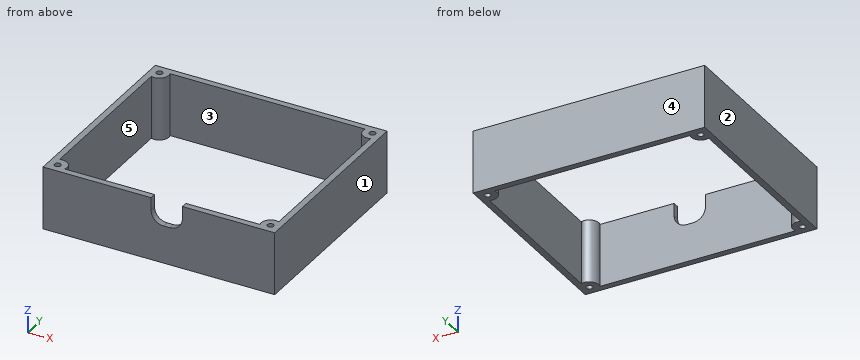
```python
from build123d import *

# Parameters (mm, degrees)
BOX010_W          = 10
BOX010_H          = 10
BOX010_DEPTH      = 10
FILLET001_R       = 4
BOX008_W          = 70
BOX008_H          = 60
BOX008_DEPTH      = 20
BOX007_W          = 74
BOX007_H          = 64
BOX007_DEPTH      = 20
CYLINDER007_R     = 1
CYLINDER007_DEPTH = 20
CYLINDER006_R     = 3
CYLINDER006_DEPTH = 20
ARRAY004_X_COUNT  = 2
ARRAY004_X_PITCH  = 68
ARRAY004_Y_COUNT  = 2
ARRAY004_Y_PITCH  = 58


with BuildPart() as fillet001:
    # Box010 → Box010 (new body)
    with BuildSketch(Plane(origin=(34.5, -4.5, 15), x_dir=(1, 0, 0), z_dir=(0, 0, 1))):
        with Locations((5, 5)):
            Rectangle(BOX010_W, BOX010_H)
    extrude(amount=BOX010_DEPTH)

    # Fillet001
    fillet001_edges = [fillet001.edges().sort_by_distance(p)[0] for p in [
        (34.5, 0.5, 15),
        (44.5, 0.5, 15),
    ]]
    fillet(fillet001_edges, radius=FILLET001_R)


with BuildPart() as wall_inner_extraction:
    # Box008 → Box008 (new body)
    with BuildSketch(Plane(origin=(2, 2, 0), x_dir=(1, 0, 0), z_dir=(0, 0, 1))):
        with Locations((35, 30)):
            Rectangle(BOX008_W, BOX008_H)
    extrude(amount=BOX008_DEPTH)


with BuildPart() as wall_box_cut:
    # Box007 → Box007 (new body)
    with BuildSketch(Plane.XY):
        with Locations((37, 32)):
            Rectangle(BOX007_W, BOX007_H)
    extrude(amount=BOX007_DEPTH)

    # Cut004: cut wall inner extraction
    add(wall_inner_extraction.part, mode=Mode.SUBTRACT)


with BuildPart() as wall_box_hole:
    # Cylinder007 → Cylinder007 (new body)
    with BuildSketch(Plane.XY):
        Circle(CYLINDER007_R)
    extrude(amount=CYLINDER007_DEPTH)


with BuildPart() as wall_fusion_cut:
    # Cylinder006 → Cylinder006 (new body)
    with BuildSketch(Plane.XY):
        Circle(CYLINDER006_R)
    extrude(amount=CYLINDER006_DEPTH)

    # Cut005: cut wall box hole
    add(wall_box_hole.part, mode=Mode.SUBTRACT)


with BuildPart() as wall_fusion_cut_1:
    # Cut005 placement: moved
    add(wall_fusion_cut.part.moved(Location((3, 3, 0))))

    # Array004 X: wall fusion cut ×2


with BuildPart() as wall_fusion_cut_2:
    add(wall_fusion_cut_1.part)
    with Locations(*[(i * ARRAY004_X_PITCH, 0, 0) for i in range(1, ARRAY004_X_COUNT)]):
        add(wall_fusion_cut_1.part)

    # Array004 Y: wall fusion cut ×2


with BuildPart() as wall_fusion_cut_3:
    add(wall_fusion_cut_2.part)
    with Locations(*[(0, i * ARRAY004_Y_PITCH, 0) for i in range(1, ARRAY004_Y_COUNT)]):
        add(wall_fusion_cut_2.part)

    # Fusion003: union wall box cut
    add(wall_box_cut.part)


with BuildPart() as wall_fusion_cut_4:
    # Fusion003 placement: moved
    add(wall_fusion_cut_3.part.moved(Location((0, 0, 3))))

    # Cut007: cut Fillet001
    add(fillet001.part, mode=Mode.SUBTRACT)


solid = wall_fusion_cut_4.part
```
Source: CAD feature listing. Evaluate the final solid. Frame: model axes, mm. Face numbers are marked on the shaded views. A direction names the side the tool comes from. Give positions to 0.01 mm unless a question says otherwise; leave off trailing zeros. Write each loop counter-clockwise with the first axis right and the second up, starting at its lowest first coordinate (ties: lowest second). Pieces come first, ordered by that corner, then holes.
1. Section query A-A (x = 16). Return the cut outline in (y, z).
2. Material intervals for line 1 along Y through (x, z) = (71, 13); line 2 along X through (y, z) = (3, 12.75); line 3 along Y through (x, z) = (22.5, 20.5), sorted ascending.
3. Section query B-B (y = 61). Return the cut outline in (x, z).
4. Access query for the marked faces 4 and 5. Directions: +Z, -Z, +X, -X, +Y, -Y. A direction counts if a zero-diameter tool reaches every point of the face in a straight line with its end or side. Return the directions, or none.
5. Pull-direction query (X, two-part tool) for the marked faces 1, 2 and 3; classes: +X half, -X half, draft (parallel to the pull), parting line (faces both ways), or undercut.
6. Section query C-C (z = 5). Return the cut outline in (x, y).
7. Section query D-D (x = 71). Return the cut outline in (y, z), then the cut area to 3 significant figures.
8. First-contact query: pin 1 (1.6 mm diameter, centred on x = 40, y = 1, fed in from +Z). Flat tip, straight axial feed; report the tip coordinate or a pass-through.
Output values:
1. outline: (0, 3) - (2, 3) - (2, 23) - (0, 23) - close; (62, 3) - (64, 3) - (64, 23) - (62, 23) - close
2. line 1: y = 0 to 2, 4 to 6, 58 to 60, 62 to 64
2. line 2: x = 0 to 2, 4 to 6, 68 to 70, 72 to 74
2. line 3: y = 0 to 2, 62 to 64
3. outline: (0, 3) - (2, 3) - (2, 23) - (0, 23) - close; (4, 3) - (6, 3) - (6, 23) - (4, 23) - close; (68, 3) - (70, 3) - (70, 23) - (68, 23) - close; (72, 3) - (74, 3) - (74, 23) - (72, 23) - close
4. face 4: +Z, -Z, +X, -X, +Y
4. face 5: +Z, -Z
5. face 1: +X half
5. face 2: -X half
5. face 3: undercut
6. outline: (0, 0) - (74, 0) - (74, 64) - (0, 64) - close; hole circle Ø2 at (3, 3); hole (2, 5.83) arc R3 cw to (5.83, 2) - (68.17, 2) arc R3 cw to (72, 5.83) - (72, 58.17) arc R3 cw to (68.17, 62) - (5.83, 62) arc R3 cw to (2, 58.17) - close; hole circle Ø2 at (3, 61); hole circle Ø2 at (71, 3); hole circle Ø2 at (71, 61)
7. outline: (0, 3) - (2, 3) - (2, 23) - (0, 23) - close; (4, 3) - (6, 3) - (6, 23) - (4, 23) - close; (58, 3) - (60, 3) - (60, 23) - (58, 23) - close; (62, 3) - (64, 3) - (64, 23) - (62, 23) - close
7. area: 160 mm2
8. pin 1: stops at z = 15.01
